```python
from build123d import *

# Parameters (mm, degrees)
IZIM1_W                     = 40
IZIM1_H                     = 15
Y_KSEKLIK_EKSTR_ZYON1_DEPTH = 10
IZIM2_R                     = 3
KES_EKSTR_ZYON1_DEPTH       = 10
IZIM4_R                     = 11.15
KES_EKSTR_ZYON2_DEPTH       = 10


with BuildPart() as part:
    # Çizim1 → Yükseklik-Ekstrüzyon1 (new body)
    with BuildSketch(Plane(origin=(0, 0, 0), x_dir=(1, 0, 0), z_dir=(0, 1, 0))):
        Rectangle(IZIM1_W, IZIM1_H)
    extrude(amount=Y_KSEKLIK_EKSTR_ZYON1_DEPTH)

    # Çizim2 → Kes-Ekstrüzyon1 (cut)
    with BuildSketch(Plane(origin=(20, 0, 0), x_dir=(0, 0, -1), z_dir=(1, 0, 0))):
        with Locations((0, 5.193163971)):
            Circle(IZIM2_R)
    extrude(amount=-KES_EKSTR_ZYON1_DEPTH, mode=Mode.SUBTRACT)

    # Çizim4 → Kes-Ekstrüzyon2 (cut)
    with BuildSketch(Plane(origin=(0, 10, 0), x_dir=(1, 0, 0), z_dir=(0, 1, 0))):
        with Locations((-8.85, -7.5)):
            Circle(IZIM4_R)
    extrude(amount=-KES_EKSTR_ZYON2_DEPTH, mode=Mode.SUBTRACT)


solid = part.part
```
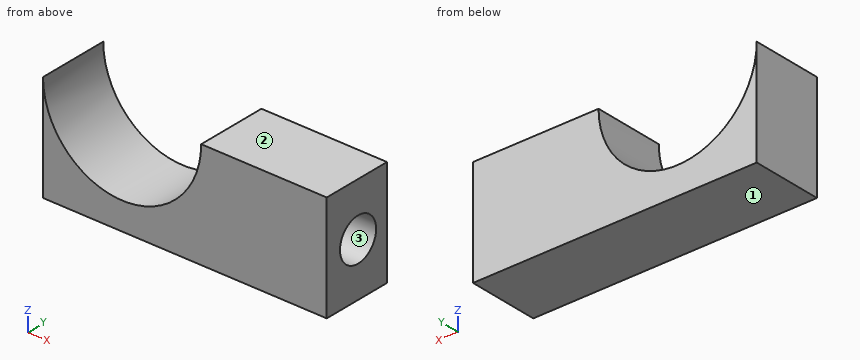
The listing builds one solid part. Answer for the finished solid, in the listing's coordinates (mm). Face numbers are marked on the shaded views. Round coordinates to 2 decimals unless told otherwise and drop trailing zeros. Loops run counter-clockwise (first coordinate to the right, second up) from the corner with the lowest first, then second, coordinate; pieces in that order, holes last. Notation, with made-up numbers: (66.25, 86.5) -> (83.25, 86.5) arc R29 cw to (83.25, 121.5) -> close; hole circle Ø2 at (29.5, 59.5). An arc over 180 degrees is marked (long way). Use one line per item in the form item = value.
1. The part is cut by section A-A on z = 2. Determine the outline of the cut face in (x, y), and give its area (3 significant figures).
Answer key:
outline = (-20, 0) -> (-18.55, 0) -> (-18.55, 10) -> (-20, 10) -> close; (0.85, 0) -> (20, 0) -> (20, 2.96) -> (10, 2.96) -> (10, 7.43) -> (20, 7.43) -> (20, 10) -> (0.85, 10) -> close
area = 161 mm²
2. For a pull along Z with two mould halves and no side action, classify the marked faces 1, 2 and 3 as released by +Z, released by -Z, zero draft, split by the parting line, or undercut.
Answer key:
face_1 = released by -Z
face_2 = released by +Z
face_3 = undercut
3. The part is cut by section D-D on z = -2.5. Determine the outline of the cut face in (x, y), and give its area (3 significant figures).
Answer key:
outline = (-20, 0) -> (-13.78, 0) -> (-13.78, 10) -> (-20, 10) -> close; (-3.92, 0) -> (20, 0) -> (20, 3.53) -> (10, 3.53) -> (10, 6.85) -> (20, 6.85) -> (20, 10) -> (-3.92, 10) -> close
area = 268 mm²
4. Find the intervals of material crossed by probe 1 along Y at (x, z) = (17, 0); probe 2 along Z at (x, y) = (16.5, 3.5); probe 3 along Z at (x, y) = (-8.5, 7), in increasing order. Write a range as [from, to].
Answer key:
probe_1 = [0, 2.19], [8.19, 10]
probe_2 = [-7.5, -2.48], [2.48, 7.5]
probe_3 = [-7.5, -3.64]
5. The part is cut by section B-B on y = 3.5. Determine the outline of the cut face in (x, z), and give its area (3 significant figures).
Answer key:
outline = (-20, -7.5) -> (20, -7.5) -> (20, -2.48) -> (10, -2.48) -> (10, 2.48) -> (20, 2.48) -> (20, 7.5) -> (2.3, 7.5) arc R11.15 cw to (-20, 7.5) -> close
area = 355 mm²
6. A flat-ended cylindrical pin translates along its axis: pin 1 Ø5 at (y, z) = (6, -1.5) entering from +X. Find the tip coordinate at first contact, or state that the pin passes through.
Answer key:
pin_1 = 20
7. The part is cut by section C-C on x = 13. Determine the outline of the cut face in (y, z).
Answer key:
outline = (0, -7.5) -> (10, -7.5) -> (10, 7.5) -> (0, 7.5) -> close; hole circle Ø6 at (5.19, 0)
